Here's how the part is built. I have some questions about the finished solid (model axes, mm). Face numbers are marked on the shaded views. A direction names the side the tool comes from. Coordinates: 2 decimals unless noted, no trailing zeros. Write each loop counter-clockwise with the first axis right and the second up, starting at its lowest first coordinate (ties: lowest second). Pieces come first, ordered by that corner, then holes. Notation, with made-up numbers: M -25.75,51 L 31.25,51 A28 cw 31.25,71 Z; hole C 63,46.25 d1. An arc over 180 degrees is marked long. Use one line per item in the form item = value. Start each with the question number.
1. I want a section at C-C, the plane x = 6.35. List the corners of the cut face in (y, z) for me (3 decimals).
2. I'm going to push flat-ended pins straight in: pin 1 Ø1 at (y, z) = (-1.5, 4.5) entering from +X; pin 2 Ø1 at (y, z) = (1, 2.5) entering from +X; pin 3 Ø3 at (x, z) = (1, 1.5) entering from -Y. Where does each tip first touch, or does it pass through?
3. Please list where these lines run through material, in increasing order: line 1 along Z through (x, y) = (-5.75, 2); line 2 along X through (y, z) = (-0.75, 5); line 3 along X through (y, z) = (-0.5, 2). Write a range as [from, to].
4. I want a section at A-A, the plane y = 0. List the corners of the cut face in (x, z) for me (3 decimals).
5. I want a section at B-B, the plane y = 2.5. List the corners of the cut face in (x, z) for me.
6. Thinking about a two-plate mould opening in X: for the marked faces 3 and 4, which applies, released by +X, released by -X, zero draft, split by the parting line, or undercut?
7. I want a section at D-D, the plane z = 4.25. List the corners of the cut face in (x, y) for me, plus the area to 3 significant figures.
8. On a 3-axis mill with a long thin cutter (end or side, diameter ignored), from which of +Z, -Z, +X, -X, +Y, -Y can I reach the whole of each face in a straight line? I mean the marked faces 1 and 2. Say none if no direction works.
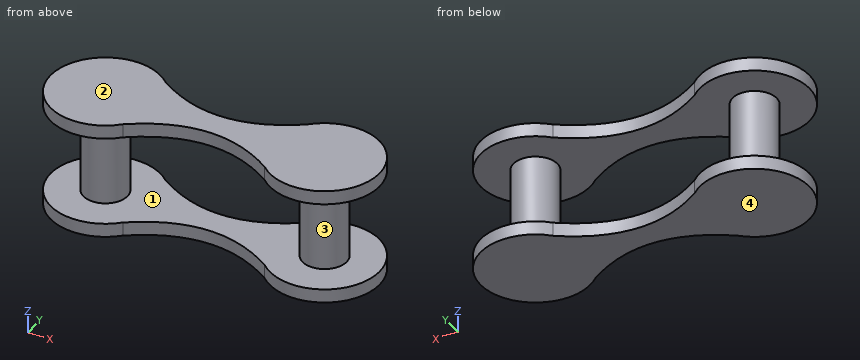
from build123d import *

# Parameters (mm, degrees)
BOSS_EXTRUDE1_DEPTH = 0.79375
SKETCH2_R           = 1.275343429
BOSS_EXTRUDE2_DEPTH = 5.159375


with BuildPart() as part:
    # Sketch1 → Boss-Extrude1 (new body)
    with BuildSketch(Plane.XY):
        with BuildLine():
            ThreePointArc((-4.10493597, 2.24506403), (-9.525, 0), (-4.10493597, -2.24506403))
            add(Edge.make_bspline(
                [(-4.10493597, -2.24506403), (0, 0.65756403), (4.10493597, -2.24506403)],
                knots=[0, 0, 0, 1, 1, 1], degree=2))
            ThreePointArc((4.10493597, -2.24506403), (9.525, 0), (4.10493597, 2.24506403))
            add(Edge.make_bspline(
                [(-4.10493597, 2.24506403), (0, -0.65756403), (4.10493597, 2.24506403)],
                knots=[0, 0, 0, 1, 1, 1], degree=2))
        make_face()
    boss_extrude1 = extrude(amount=BOSS_EXTRUDE1_DEPTH)

    # Sketch2 → Boss-Extrude2 (add)
    with BuildSketch(Plane.XY.offset(0.79375)):
        with Locations((-6.35, 0)):
            Circle(SKETCH2_R)
        with Locations(Location((6.35, 0, 0), (0, 0, 180))):
            Circle(SKETCH2_R)
    extrude(amount=BOSS_EXTRUDE2_DEPTH)

    # Mirror1: Boss-Extrude1 across plane
    add(boss_extrude1.mirror(Plane.XY.offset(3.3734375)))


solid = part.part
Answer list:
q1.outline = M -3.175,0 L 3.175,0 L 3.175,0.794 L 1.275,0.794 L 1.275,5.953 L 3.175,5.953 L 3.175,6.747 L -3.175,6.747 L -3.175,5.953 L -1.275,5.953 L -1.275,0.794 L -3.175,0.794 Z
q2.pin_1 = 7.14
q2.pin_2 = 7.52
q2.pin_3 = -1.26
q3.line_1 = [0, 0.79], [5.95, 6.75]
q3.line_2 = [-7.38, -5.32], [5.32, 7.38]
q3.line_3 = [-7.52, -5.18], [5.18, 7.52]
q4.outline = M -9.525,0 L 9.525,0 L 9.525,0.794 L 7.625,0.794 L 7.625,5.953 L 9.525,5.953 L 9.525,6.747 L -9.525,6.747 L -9.525,5.953 L -7.625,5.953 L -7.625,0.794 L -9.525,0.794 Z; hole M -5.075,0.794 L 5.075,0.794 L 5.075,5.953 L -5.075,5.953 Z
q5.outline = M -8.31,0 L -4.39,0 L -4.39,0.79 L -8.31,0.79 Z; M -8.31,5.95 L -4.39,5.95 L -4.39,6.75 L -8.31,6.75 Z; M 4.39,0 L 8.31,0 L 8.31,0.79 L 4.39,0.79 Z; M 4.39,5.95 L 8.31,5.95 L 8.31,6.75 L 4.39,6.75 Z
q6.face_3 = undercut
q6.face_4 = zero draft
q7.outline = C -6.35,0 d2.55; C 6.35,0 d2.55
q7.area = 10.2 mm²
q8.face_1 = none
q8.face_2 = +Z, +X, -X, +Y, -Y
